Verification items for the finished model (mm, model axes). Coordinates: 2 decimals unless noted, no trailing zeros. Write each loop counter-clockwise with the first axis right and the second up, starting at its lowest first coordinate (ties: lowest second). Pieces come first, ordered by that corner, then holes. Notation, with made-up numbers: (0, 87.5) -> (48, 87.5) arc R22 ccw to (48, 123.5) -> close; hole circle Ø7 at (-21, 12.5). An arc over 180 degrees is marked (long way). Answer in a Markdown table with one row per item.
```python
from build123d import *

# Parameters (mm, degrees)
F0_R     = 12.7
F0_R_2   = 12.827
F1_DEPTH = 11.938
F3_DEPTH = 25.4
F5_DEPTH = 25.4


with BuildPart() as f1:
    # F0 (on Top) → F1 (new body)
    with BuildSketch(Plane.XY):
        with BuildLine():
            Line((58.34362, -61.556164), (72.2663, -53.5179))
            ThreePointArc((72.2663, -53.5179), (76.738749, -51.665351), (81.538278, -51.033481))
            Line((81.538278, -51.033481), (174.210487, -51.033481))
            ThreePointArc((174.210487, -51.033481), (179.010016, -51.665351), (183.482465, -53.517901))
            Line((183.482465, -53.517901), (197.405145, -61.556163))
            ThreePointArc((197.405145, -61.556163), (201.877594, -63.408713), (206.677123, -64.040582))
            Line((206.677123, -64.040582), (427.024152, -64.040582))
            ThreePointArc((427.024152, -64.040582), (438.226145, -60.274774), (444.878456, -50.506831))
            Line((444.878456, -50.506831), (458.014524, -3.695302))
            ThreePointArc((458.014524, -3.695302), (458.530955, -1.213822), (458.704177, 1.314901))
            Line((458.704177, 1.314901), (458.704177, 19.696639))
            Line((458.704177, 19.696639), (458.704177, 281.824639))
            Line((458.704177, 281.824639), (458.704177, 300.206376))
            ThreePointArc((458.704177, 300.206376), (458.530955, 302.735101), (458.014524, 305.216583))
            Line((458.014524, 305.216583), (444.878456, 352.02811))
            ThreePointArc((444.878456, 352.02811), (438.226145, 361.796053), (427.024152, 365.561861))
            Line((427.024152, 365.561861), (206.677126, 365.561861))
            ThreePointArc((206.677126, 365.561861), (201.877596, 364.929991), (197.405147, 363.077442))
            Line((197.405147, 363.077442), (183.482464, 355.039177))
            ThreePointArc((183.482464, 355.039177), (179.010015, 353.186628), (174.210486, 352.554758))
            Line((174.210486, 352.554758), (81.538278, 352.554758))
            ThreePointArc((81.538278, 352.554758), (76.738749, 353.186628), (72.2663, 355.039177))
            Line((72.2663, 355.039177), (58.34362, 363.07744))
            ThreePointArc((58.34362, 363.07744), (53.871171, 364.929989), (49.071641, 365.561859))
            Line((49.071641, 365.561859), (-185.331903, 365.561859))
            ThreePointArc((-185.331903, 365.561859), (-191.289303, 367.091944), (-195.772045, 371.30345))
            ThreePointArc((-195.772045, 371.30345), (-217.185472, 381.121689), (-234.872313, 365.561859))
            Line((-234.872313, 365.561859), (-251.80617, 305.216581))
            ThreePointArc((-251.80617, 305.216581), (-252.322601, 302.735099), (-252.495823, 300.206375))
            Line((-252.495823, 300.206375), (-252.495823, 281.82464))
            Line((-252.495823, 281.82464), (-252.495823, 19.69664))
            Line((-252.495823, 19.69664), (-252.495823, 1.314901))
            ThreePointArc((-252.495823, 1.314901), (-252.322601, -1.213823), (-251.80617, -3.695304))
            Line((-251.80617, -3.695304), (-234.872313, -64.040583))
            ThreePointArc((-234.872313, -64.040583), (-217.185472, -79.600413), (-195.772045, -69.782174))
            ThreePointArc((-195.772045, -69.782174), (-191.289303, -65.570667), (-185.331903, -64.040583))
            Line((-185.331903, -64.040583), (49.071641, -64.040583))
            ThreePointArc((49.071641, -64.040583), (53.871171, -63.408713), (58.34362, -61.556164))
        make_face()
        with Locations((-85.085704, 150.760638)):
            Circle(F0_R, mode=Mode.SUBTRACT)
        with Locations((197.19935, -12.218626)):
            Circle(F0_R_2, mode=Mode.SUBTRACT)
        with Locations((103.105436, 150.760638)):
            Circle(F0_R_2, mode=Mode.SUBTRACT)
        with Locations((197.19935, 313.739902)):
            Circle(F0_R_2, mode=Mode.SUBTRACT)
    extrude(amount=F1_DEPTH)

    # F2 (on face) → F3 (cut)
    with BuildSketch(Plane.XY.offset(11.938)):
        Polygon((-170.314763, 272.426638), (-185.808763, 272.426638), (-188.983763, 272.426638), (-188.983763, 259.472638), (-185.808763, 259.472638), (-170.314763, 259.472638), (-167.139763, 259.472638), (-167.139763, 272.426638), align=None)
        Polygon((-136.608963, 259.472638), (-121.114963, 259.472638), (-117.939963, 259.472638), (-117.939963, 272.426638), (-121.114963, 272.426638), (-136.608963, 272.426638), (-139.783963, 272.426638), (-139.783963, 259.472638), align=None)
        Polygon((-188.983763, 29.094638), (-185.808763, 29.094638), (-170.314763, 29.094638), (-167.139763, 29.094638), (-167.139763, 42.048638), (-170.314763, 42.048638), (-185.808763, 42.048638), (-188.983763, 42.048638), align=None)
        Polygon((-117.939963, 42.048638), (-121.114963, 42.048638), (-136.608963, 42.048638), (-139.783963, 42.048638), (-139.783963, 29.094638), (-136.608963, 29.094638), (-121.114963, 29.094638), (-117.939963, 29.094638), align=None)
    extrude(amount=-F3_DEPTH, mode=Mode.SUBTRACT)

    # F4 (on face) → F5 (cut)
    with BuildSketch(Plane.XY.offset(11.938)):
        Polygon((31.031037, 73.671638), (-20.022963, 73.671638), (-23.197963, 73.671638), (-23.197963, 60.717638), (-20.022963, 60.717638), (31.031037, 60.717638), (34.206037, 60.717638), (34.206037, 73.671638), align=None)
        Polygon((187.368037, 73.671638), (184.193037, 73.671638), (133.139037, 73.671638), (129.964037, 73.671638), (129.964037, 60.717638), (133.139037, 60.717638), (184.193037, 60.717638), (187.368037, 60.717638), align=None)
        Polygon((-23.197963, 226.071638), (-20.022963, 226.071638), (31.031037, 226.071638), (34.206037, 226.071638), (34.206037, 239.025638), (31.031037, 239.025638), (-20.022963, 239.025638), (-23.197963, 239.025638), align=None)
        Polygon((133.139037, 226.071638), (184.193037, 226.071638), (187.368037, 226.071638), (187.368037, 239.025638), (184.193037, 239.025638), (133.139037, 239.025638), (129.964037, 239.025638), (129.964037, 226.071638), align=None)
    extrude(amount=-F5_DEPTH, mode=Mode.SUBTRACT)


solid = f1.part
```
1. Section check D-D, the plane z = 9. State how many separate pieces and enclosed holes the cut face has, plus the area to 3 significant figures.
Geometry says:
| item | result |
|---|---|
| separate pieces | 1 |
| enclosed holes | 12 |
| area | 295,000 mm^2 |
2. Mould release check, pull along X, two halves, no side actions. Record for faces 1 (the cylindrical face through (184.385, -11.655, 5.885)), 2 (the cylindrical face through (438.36, 361.694, 5.885)), 3 (the flat face through (98, 103, 11.938)): released by +X, released by -X, zero draft, split by the parting line, or undercut.
Geometry says:
| item | result |
|---|---|
| face 1 | undercut |
| face 2 | released by +X |
| face 3 | zero draft |
3. Section check C-C, the plane x = 289.5. Record the boundary of the cut face in (y, z), plus the area to 3 significant figures.
Geometry says:
| item | result |
|---|---|
| outline | (-64.04, 0) -> (365.56, 0) -> (365.56, 11.94) -> (-64.04, 11.94) -> close |
| area | 5,130 mm^2 |
4. Section check B-B, the plane x = 140. Record the boundary of the cut face in (y, z), plus the area to 3 significant figures.
Geometry says:
| item | result |
|---|---|
| outline | (-51.03, 0) -> (60.72, 0) -> (60.72, 11.94) -> (-51.03, 11.94) -> close; (73.67, 0) -> (226.07, 0) -> (226.07, 11.94) -> (73.67, 11.94) -> close; (239.03, 0) -> (352.55, 0) -> (352.55, 11.94) -> (239.03, 11.94) -> close |
| area | 4,510 mm^2 |
5. Section check A-A, the plane x = -4. Record the boundary of the cut face in (y, z).
Geometry says:
| item | result |
|---|---|
| outline | (-64.04, 0) -> (60.72, 0) -> (60.72, 11.94) -> (-64.04, 11.94) -> close; (73.67, 0) -> (226.07, 0) -> (226.07, 11.94) -> (73.67, 11.94) -> close; (239.03, 0) -> (365.56, 0) -> (365.56, 11.94) -> (239.03, 11.94) -> close |
6. Thickness scan on line 1 (Y direction, x = -185, z = 5.75); line 2 (X direction, y = 237.5, z = 3.5); line 3 (Y direction, x = 15.5, z = 5). Record the ranges inside material, lowest first. Write a range as from..to.
Geometry says:
| item | result |
|---|---|
| line 1 | -64.04..29.09, 42.05..259.47, 272.43..365.56 |
| line 2 | -252.5..-23.2, 34.21..129.96, 187.37..458.7 |
| line 3 | -64.04..60.72, 73.67..226.07, 239.03..365.56 |
7. Depth check by flat-ended pin: P1, Ø3, axis at y = -13, z = 6.5, coming from the +X side; P2, Ø4, axis at x = 48, z = 4, coming from the +Y side; P3, Ø3.5, axis at x = -128.5, z = 3.5, coming from the -Y side; P4, Ø10, axis at x = 0.5, y = 229, coming from the -Z side. Enter the tip coordinate at first touch or a pass-through.
Geometry says:
| item | result |
|---|---|
| P1 | x = 455.82 |
| P2 | y = 365.56 |
| P3 | y = -64.04 |
| P4 | z = 0 |
